The figure shows three views and two pictorial views of one solid part (mm, origin at its lowest corner). Answer the questions. A direction names the side the tool comes from. Give positions to 0.01 mm unless a question says otherwise; leave off trailing zeros. Write each loop counter-clockwise with the first axis right and the second up, starting at its lowest first coordinate (ties: lowest second). Pieces come first, ordered by that corner, then holes. Notation, with made-up numbers: (40, 36.5) - (60, 36.5) arc R21 ccw to (60, 48.5) - close; hole circle Ø9 at (3, 50.25). An arc over 180 degrees is marked (long way). Use CSV: the item, a comma, the result in double quotes. Start each with the question number.
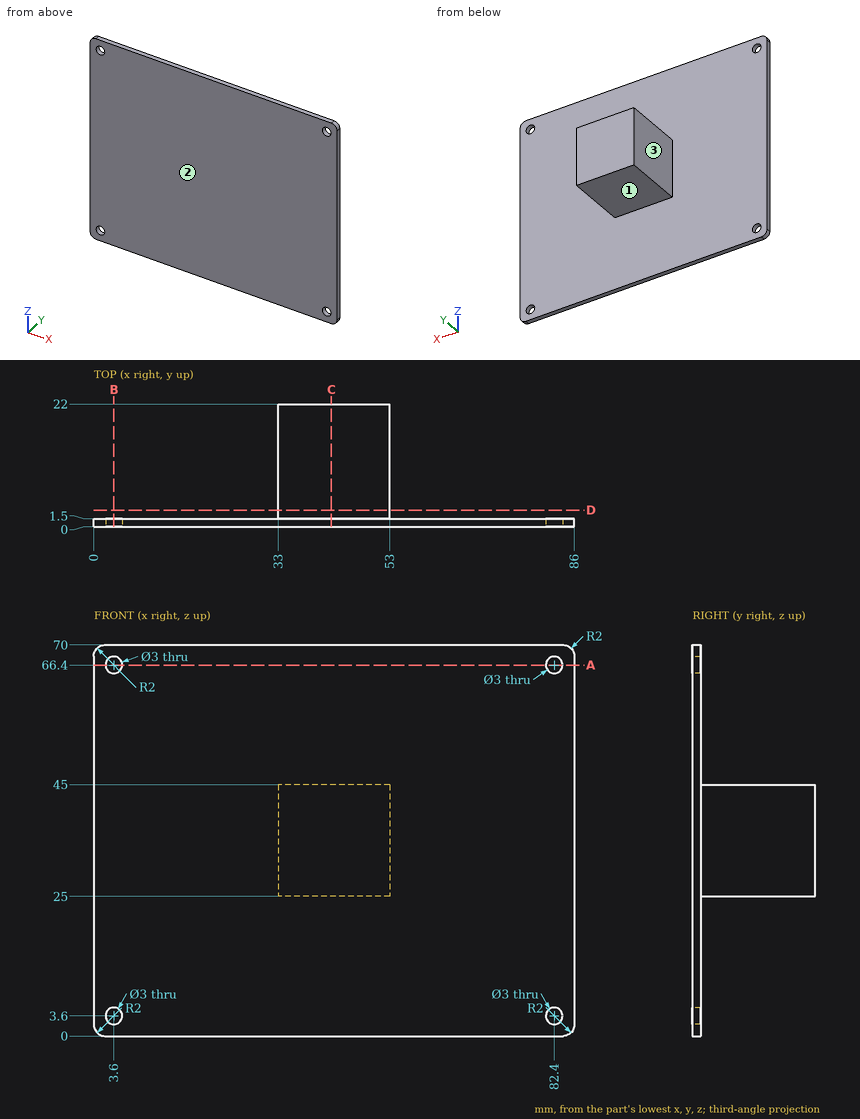
(1) Which of the six approach directions +Z, -Z, +X, -X, +Y, -Y give full straight-line access (tool end or side, diameter ignored) to the marked faces 1, 2 and 3?
(2) Given P1, Ø4, axis at y = 15.5, z = 25.5, coming from the +X side; P2, Ø5, axis at y = 13.5, z = 23.5, coming from the -X side; P3, Ø3.5, axis at x = 82.4, z = 3.6, coming from the -Y side; P4, Ø4, axis at x = 3.6, z = 3.6, coming from the +Y side, each flat-ended and moving along its own axis, determine where each tip first touches the part or whether it passes through.
(3) The part is cut by section D-D on y = 3. Write down the section's boundary in (x, z), plus the area to 3 significant figures.
(4) The part is cut by section A-A on z = 66.4. Write down the section's boundary in (x, y), plus the area to 3 significant figures.
(5) Consider probe 1 along X at (y, z) = (0.65, 3.6); probe 2 along Y at (x, z) = (44, 18.5); probe 3 along Z at (x, y) = (50.5, 19.25). Determine where each line is inside the solid, lowest interval first.
(6) The part is cut by section B-B on x = 3.6. Write down the section's boundary in (y, z), plus the area to 3 significant figures.
(7) The part is cut by section C-C on x = 42.5. Write down the section's boundary in (y, z), plus the area to 3 significant figures.
Reported:
1,face 1,"-Z, +X, -X, +Y"
1,face 2,"+Z, -Z, +X, -X, -Y"
1,face 3,"+Z, -Z, -X, +Y"
2,P1,"x = 53"
2,P2,"x = 33"
2,P3,"y = 0"
2,P4,"y = 1.5"
3,outline,"(33, 25) - (53, 25) - (53, 45) - (33, 45) - close"
3,area,"400 mm²"
4,outline,"(0, 0) - (2.1, 0) - (2.1, 1.5) - (0, 1.5) - close; (5.1, 0) - (80.9, 0) - (80.9, 1.5) - (5.1, 1.5) - close; (83.9, 0) - (86, 0) - (86, 1.5) - (83.9, 1.5) - close"
4,area,"120 mm²"
5,probe 1,"0 to 2.1, 5.1 to 80.9, 83.9 to 86"
5,probe 2,"0 to 1.5"
5,probe 3,"25 to 45"
6,outline,"(0, 0) - (1.5, 0) - (1.5, 2.1) - (0, 2.1) - close; (0, 5.1) - (1.5, 5.1) - (1.5, 64.9) - (0, 64.9) - close; (0, 67.9) - (1.5, 67.9) - (1.5, 70) - (0, 70) - close"
6,area,"96.0 mm²"
7,outline,"(0, 0) - (1.5, 0) - (1.5, 25) - (22, 25) - (22, 45) - (1.5, 45) - (1.5, 70) - (0, 70) - close"
7,area,"515 mm²"
